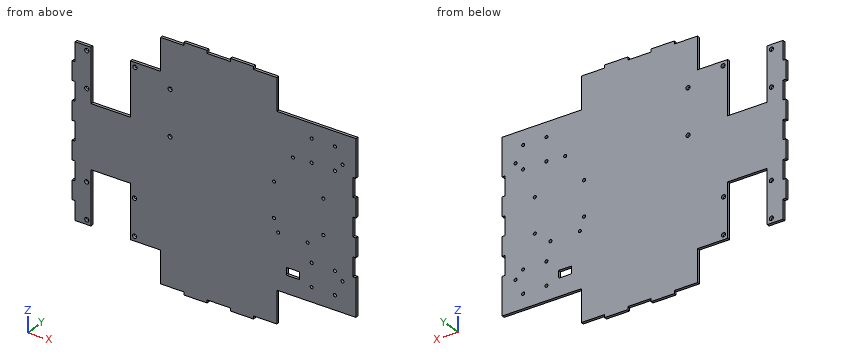
from build123d import *

# Parameters (mm, degrees)
SKETCH1_R           = 1.65
SKETCH1_R_2         = 2.25
BOSS_EXTRUDE1_DEPTH = 3


with BuildPart() as part:
    # Sketch1 → Boss-Extrude1 (new body)
    with BuildSketch(Plane(origin=(0, 0, 0), x_dir=(1, 0, 0), z_dir=(0, 1, 0))):
        Polygon((152.5, 92), (67.5, 92), (67.5, 126.825), (42.5, 126.825), (42.5, 130), (17.5, 130), (17.5, 126.825), (-7.5, 126.825), (-7.5, 130), (-32.5, 130), (-32.5, 126.825), (-57.5, 126.825), (-57.5, 92), (-90.0007, 92), (-90.0007, 34), (-132.3969, 34), (-132.3969, 92), (-149.325, 92), (-149.325, 71.555555556), (-152.5, 71.555555556), (-152.5, 51.111111111), (-149.325, 51.111111111), (-149.325, 30.666666667), (-152.5, 30.666666667), (-152.5, 10.222222222), (-149.325, 10.222222222), (-149.325, -10.222222222), (-152.5, -10.222222222), (-152.5, -30.666666667), (-149.325, -30.666666667), (-149.325, -51.111111111), (-152.5, -51.111111111), (-152.5, -71.555555556), (-149.325, -71.555555556), (-149.325, -92), (-132.3969, -92), (-132.3969, -34), (-90.0007, -34), (-90.0007, -92), (-57.5, -92), (-57.5, -126.825), (-32.5, -126.825), (-32.5, -130), (-7.5, -130), (-7.5, -126.825), (17.5, -126.825), (17.5, -130), (42.5, -130), (42.5, -126.825), (67.5, -126.825), (67.5, -92), (152.5, -92), (152.5, -51.111111111), (149.325, -51.111111111), (149.325, -30.666666667), (152.5, -30.666666667), (152.5, -10.222222222), (149.325, -10.222222222), (149.325, 10.222222222), (152.5, 10.222222222), (152.5, 30.666666667), (149.325, 30.666666667), (149.325, 51.111111111), (152.5, 51.111111111), align=None)
        with Locations((105, 76.5)):
            Circle(SKETCH1_R, mode=Mode.SUBTRACT)
        with Locations((130, 76.5)):
            Circle(SKETCH1_R, mode=Mode.SUBTRACT)
        with Locations((-136.8894, -87)):
            Circle(SKETCH1_R_2, mode=Mode.SUBTRACT)
        with Locations((-85.0006, -87)):
            Circle(SKETCH1_R_2, mode=Mode.SUBTRACT)
        with Locations((-47.3083, -77)):
            Circle(SKETCH1_R_2, mode=Mode.SUBTRACT)
        with Locations((-136.8894, -48)):
            Circle(SKETCH1_R_2, mode=Mode.SUBTRACT)
        with Locations((-47.3083, -28)):
            Circle(SKETCH1_R_2, mode=Mode.SUBTRACT)
        with Locations((105, -76.5)):
            Circle(SKETCH1_R, mode=Mode.SUBTRACT)
        with Locations((130, -76.5)):
            Circle(SKETCH1_R, mode=Mode.SUBTRACT)
        with Locations((84.82, -50.289)):
            Circle(SKETCH1_R, mode=Mode.SUBTRACT)
        with Locations((105, -51.5)):
            Circle(SKETCH1_R, mode=Mode.SUBTRACT)
        with Locations((130, -51.5)):
            Circle(SKETCH1_R, mode=Mode.SUBTRACT)
        with Locations((138.16, -60.452)):
            Circle(SKETCH1_R, mode=Mode.SUBTRACT)
        with Locations((64.5, -18.75)):
            Circle(SKETCH1_R, mode=Mode.SUBTRACT)
        with Locations((117.5, -18.75)):
            Circle(SKETCH1_R, mode=Mode.SUBTRACT)
        with Locations((-136.88945, 48)):
            Circle(SKETCH1_R_2, mode=Mode.SUBTRACT)
        with Locations((-85.50815, 48)):
            Circle(SKETCH1_R_2, mode=Mode.SUBTRACT)
        with Locations((-136.88945, 87)):
            Circle(SKETCH1_R_2, mode=Mode.SUBTRACT)
        with Locations((-85.50815, 87)):
            Circle(SKETCH1_R_2, mode=Mode.SUBTRACT)
        with Locations((64.5, 18.75)):
            Circle(SKETCH1_R, mode=Mode.SUBTRACT)
        with Locations((68.945, 32.131)):
            Circle(SKETCH1_R, mode=Mode.SUBTRACT)
        with Locations((100.695, 32.131)):
            Circle(SKETCH1_R, mode=Mode.SUBTRACT)
        with Locations((117.5, 18.75)):
            Circle(SKETCH1_R, mode=Mode.SUBTRACT)
        with Locations((105, 51.5)):
            Circle(SKETCH1_R, mode=Mode.SUBTRACT)
        with Locations((130, 51.5)):
            Circle(SKETCH1_R, mode=Mode.SUBTRACT)
        with Locations((138.16, 59.563)):
            Circle(SKETCH1_R, mode=Mode.SUBTRACT)
        with BuildLine():
            Line((91.88, 65.143), (77.88, 65.143))
            Line((77.88, 65.143), (77.88, 72.143))
            ThreePointArc((77.88, 72.143), (78.172893219, 72.850106781), (78.88, 73.143))
            Line((78.88, 73.143), (90.88, 73.143))
            ThreePointArc((90.88, 73.143), (91.587106781, 72.850106781), (91.88, 72.143))
            Line((91.88, 72.143), (91.88, 65.143))
        make_face(mode=Mode.SUBTRACT)
    extrude(amount=BOSS_EXTRUDE1_DEPTH)


solid = part.part
Work out the finished part from the listing and answer in its coordinate system (mm). Give positions to 0.01 mm unless a question says otherwise; leave off trailing zeros. Write each loop counter-clockwise with the first axis right and the second up, starting at its lowest first coordinate (ties: lowest second). Pieces come first, ordered by that corner, then holes. Notation, with made-up numbers: (-27.5, 21.5) - (15.5, 21.5) arc R22 ccw to (15.5, 42.5) - close; hole circle Ø10 at (-40, -28). An arc over 180 degrees is marked (long way). One line per item, written item: value. Start each with the question number.
1. Find section B-B (z = 97.5). Write down the section's boundary in (x, y).
2. Given pin 1 (4 mm diameter, centred on x = 105, z = 76.5, fed in from -Y); pin 2 (0.9 mm diameter, centred on x = 10, y = 1, fed in from +Z) (3 decimals); pin 3 (1.5 mm diameter, centred on y = 2, z = 114, fed in from -X), each flat-ended and moving along its own axis, determine where each tip first touches the part or whether it passes through.
3. Find section D-D (z = -4). Write down the section's boundary in (x, y) (3 decimals), then the cut area to 3 significant figures.
4. Find section C-C (y = 2.5). State how many separate pieces and enclosed holes the cut face has, then the cut area to 3 significant figures.
5. Find section A-A (z = 42). Write down the section's boundary in (x, y) (3 decimals).
6. Consider probe 1 along Z at (x, y) = (105, 0.85); probe 2 along X at (y, z) = (0.35, -72.5) (3 decimals); probe 3 along X at (y, z) = (1.85, -51.5). Determine where each line is inside the solid, lowest interval first.
Geometry results:
1. outline: (-57.5, 0) - (67.5, 0) - (67.5, 3) - (-57.5, 3) - close
2. pin 1: y = 0
2. pin 2: z = 126.825
2. pin 3: x = -57.5
3. outline: (-149.325, 0) - (149.325, 0) - (149.325, 3) - (-149.325, 3) - close
3. area: 896 mm2
4. separate pieces: 1
4. enclosed holes: 27
4. area: 59,300 mm2
5. outline: (-149.325, 0) - (-132.397, 0) - (-132.397, 3) - (-149.325, 3) - close; (-90.001, 0) - (149.325, 0) - (149.325, 3) - (-90.001, 3) - close
6. probe 1: -92 to -78.15, -74.85 to -53.15, -49.85 to 49.85, 53.15 to 74.85, 78.15 to 92
6. probe 2: -149.325 to -132.397, -90.001 to 77.946, 91.814 to 152.5
6. probe 3: -152.5 to -132.4, -90 to 103.35, 106.65 to 128.35, 131.65 to 152.5
